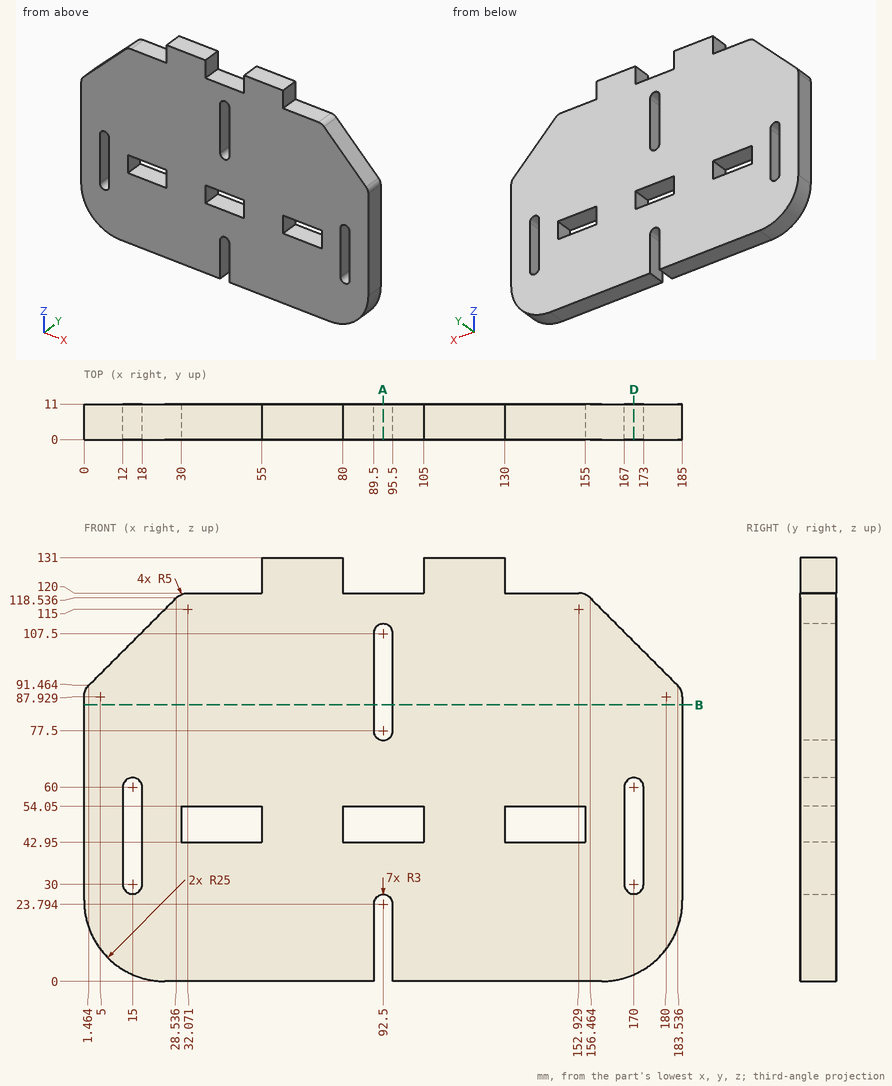
Print and shaded views of the part. All mm, measured from the part's lowest x, y and z. Give positions to 0.01 mm unless a question says otherwise; leave off trailing zeros. Loops run counter-clockwise (first coordinate to the right, second up) from the corner with the lowest first, then second, coordinate; pieces in that order, holes last. Notation, with made-up numbers: (56.5, 16.5) -> (101.5, 16.5) arc R29 ccw to (101.5, 48.5) -> close; hole circle Ø6 at (-34, 72). An arc over 180 degrees is marked (long way). Use CSV: the item, a comma, the result in double quotes. Start each with the question number.
1) Wall check: line 1 (X direction, y = 4.5, z = 44); line 2 (X direction, y = 4.25, z = 30); line 3 (Z direction, x = 42.5, y = 1.5). Give the ranges that are in metal, low to high.
2) Slice it at B-B on z = 85.5. Give the cut face in (x, y).
3) Flat gauge pins, fed straight in: pin 1 Ø5.5 at (y, z) = (8, 15) entering from +X (1 decimal); pin 2 Ø5.5 at (x, y) = (45, 6) entering from +Z; pin 3 Ø3.5 at (y, z) = (4, 127.5) entering from +X. Where does each tip first touch, or does it go through?
4) Slice it at D-D on x = 170. Give the cut face in (y, z), plus the area to 3 significant figures.
5) Slice it at A-A on x = 92.5. Give the number of separate pieces and of enclosed holes in the cut face, plus the area to 3 significant figures.
Computed values:
1,line 1,"x = 0 to 12, 18 to 30, 55 to 80, 105 to 130, 155 to 167, 173 to 185"
1,line 2,"x = 0 to 12, 18 to 167, 173 to 185"
1,line 3,"z = 0 to 42.95, 54.05 to 120"
2,outline,"(0, 0) -> (89.5, 0) -> (89.5, 11) -> (0, 11) -> close; (95.5, 0) -> (185, 0) -> (185, 11) -> (95.5, 11) -> close"
3,pin 1,"stops at x = 183.9"
3,pin 2,"stops at z = 120"
3,pin 3,"stops at x = 130"
4,outline,"(0, 2.09) -> (11, 2.09) -> (11, 27) -> (0, 27) -> close; (0, 63) -> (11, 63) -> (11, 105) -> (0, 105) -> close"
4,area,"736 mm^2"
5,separate pieces,"3"
5,enclosed holes,"0"
5,area,"507 mm^2"
